Can you work these out from the model? Positions are in its coordinate system, mm. A direction names the side the tool comes from. Coordinates: 2 decimals unless noted, no trailing zeros. Order: outer loops, then holes, each group sorted by start corner. A loop starts at its lowest first (then second) coordinate and runs counter-clockwise, first axis right, second up. Notation, with made-up numbers: (78, 57) - (124, 57) arc R7 cw to (124, 67) - close; hole circle Ø3 at (4.5, 40). An arc over 180 degrees is marked (long way). Return JSON: item names as keys, results as strings. Group by question number.
1) If we mould it in two halves opening along Z, with no side actions, what happens to faces 1 (the face through (3, 9, -292.1)), 2 (the face through (-241.3, 9, -117)), 3 (the face through (-166, 9, 63.5))? For each: pulls with the +Z half, pulls with the -Z half, needs draft (parallel to the pull), parting line crosses it, or undercut.
2) If I drill on line 1 along Z through (x, y) = (221, 13.75); line 2 along X through (y, z) = (1.5, 204.5), over which ranges is the centre line in solid material (lowest first)?
3) Imagine slicing it at A-A (x = -148). Write out the boundary of the cut face in (y, z).
4) Which directions (+Z, -Z, +X, -X, +Y, -Y) give clear straight access to the entire face, cutting with the end or side of a thin tool? Please do faces 4 (the face through (241.3, 9, 251)), 5 (the face through (166, 9, 209.55)), 6 (the face through (-164, 9, 209.55)).
5) For pin 1 Ø5 at (y, z) = (11, 108) entering from -X; pin 2 Ø5 at (x, z) = (18.5, 146) entering from -Y; pin 3 Ø2 at (y, z) = (3, 191) entering from +X, each with a flat end and sliding along its axis, tell me the tip position at first contact or that it passes through.
6) Imagine slicing it at C-C (z = 78). Write out the boundary of the cut face in (x, y), and give its area (3 significant figures).
7) Imagine slicing it at B-B (y = 8.25). Write out the boundary of the cut face in (x, z), and give its area (3 significant figures).
Autodesk Inventor part; units mm, degrees
ref_plane "XZ Plane" through (0, 0, 0) normal (0, 1, 0) x (-1, 0, 0)
ref_plane "XY Plane" through (0, 0, 0) normal (0, 0, 1) x (1, 0, 0)
sketch "Sketch1" plane through (0, 0, 0) normal (0, 1, 0) x (-1, 0, 0)
  line L0 (-241.3, 292.1) -> (-241.3, -292.1)
  line L1 (-241.3, -292.1) -> (241.3, -292.1)
  line L2 (241.3, -292.1) -> (241.3, 292.1)
  line L3 (241.3, 292.1) -> (-241.3, 292.1)
  line L4 (-241.3, 292.1) -> (241.3, -292.1) construction
  line L5 (-241.3, -292.1) -> (241.3, 292.1) construction
  point P0 (0, 0)
  dimension "baseLength" = 584.2
  dimension "baseWidth" = 482.6
extrude "Extrusion1" add sketch "Sketch1" along normal blind 17.78
sketch "Sketch2" plane through (0, 0, 0) normal (0, -1, 0) x (1, 0, 0)
  line L0 (241.3, 292.1) -> (241.3, -292.1)
  line L1 (241.3, 209.55) -> (88.9, 209.55)
  line L2 (88.9, 209.55) -> (88.9, 63.5)
  line L3 (88.9, 63.5) -> (241.3, 63.5)
  line L4 (241.3, 63.5) -> (241.3, 209.55)
  line L5 (-241.3, 292.1) -> (241.3, 292.1)
  point P0 (0, 0)
  dimension "backToEndOfGearBox" = 82.55
  dimension "backToFrontOfGearBox" = 228.6
  dimension "wdithForGearBox" = 152.4
extrude "Extrusion2" cut sketch "Sketch2" against normal through all
mirror "Mirror1" about plane through (0, 0, 0) normal (1, 0, 0) of "Extrusion2"
equation "\"spaceingAlongSides\" = 3.175"
equation "\"distanceFromBackForEndBolt\" = 38.1"
equation "\"spacingForBolt\" = 25.4"
equation "\"widthOfSpacingForBolt\" = 12.7"
equation "\"lengthOfSpacingForBolt\" = 25.4"
properties part number "RhinoBottomFloorPlate04" material "Wood (Birch)"
Calculated:
{
 "1": {"face 1": "pulls with the -Z half", "face 2": "needs draft", "face 3": "undercut"},
 "2": {"line 1": "-292.1 to 63.5, 209.55 to 292.1", "line 2": "-88.9 to 88.9"},
 "3": {"outline": "(0, -292.1) - (17.78, -292.1) - (17.78, 63.5) - (0, 63.5) - close; (0, 209.55) - (17.78, 209.55) - (17.78, 292.1) - (0, 292.1) - close"},
 "4": {"face 4": "+Z, -Z, +X, +Y, -Y", "face 5": "+X, +Y, -Y", "face 6": "-X, +Y, -Y"},
 "5": {"pin 1": "x = -88.9", "pin 2": "y = 0", "pin 3": "x = 88.9"},
 "6": {"outline": "(-88.9, 0) - (88.9, 0) - (88.9, 17.78) - (-88.9, 17.78) - close", "area": "3,160 mm2"},
 "7": {"outline": "(-241.3, -292.1) - (241.3, -292.1) - (241.3, 63.5) - (88.9, 63.5) - (88.9, 209.55) - (241.3, 209.55) - (241.3, 292.1) - (-241.3, 292.1) - (-241.3, 209.55) - (-88.9, 209.55) - (-88.9, 63.5) - (-241.3, 63.5) - close", "area": "237,000 mm2"}
}
